The listing builds one solid part. Answer for the finished solid, in the listing's coordinates (mm). Face numbers are marked on the shaded views. A direction names the side the tool comes from. Round coordinates to 2 decimals unless told otherwise and drop trailing zeros. Order: outer loops, then holes, each group sorted by start corner. A loop starts at its lowest first (then second) coordinate and runs counter-clockwise, first axis right, second up. Notation, with made-up numbers: (42, 60) - (85, 60) arc R23 cw to (85, 95) - close; hole circle Ø5 at (44.5, 24). An arc over 180 degrees is marked (long way). Write item = value, one per line.
from build123d import *

# Parameters (mm, degrees)
SKETCH1_W           = 50
SKETCH1_H           = 25
BOSS_EXTRUDE1_DEPTH = 6
SKETCH2_R           = 1
SKETCH2_R_2         = 0.999812185
CUT_EXTRUDE1_DEPTH  = 6
CUT_EXTRUDE2_DEPTH  = 6
FILLET1_R           = 2


with BuildPart() as part:
    # Sketch1 → Boss-Extrude1 (new body)
    with BuildSketch(Plane(origin=(0, 0, 0), x_dir=(1, 0, 0), z_dir=(0, 1, 0))):
        Rectangle(SKETCH1_W, SKETCH1_H)
    extrude(amount=BOSS_EXTRUDE1_DEPTH)

    # Sketch2 → Cut-Extrude1 (cut)
    with BuildSketch(Plane(origin=(0, 0, 0), x_dir=(1, 0, 0), z_dir=(0, 1, 0))):
        with Locations((-21, 8.5)):
            Circle(SKETCH2_R)
        with Locations((21, 8.5)):
            Circle(SKETCH2_R_2)
        with Locations((-21, -8.5)):
            Circle(SKETCH2_R)
        with Locations((21, -8.5)):
            Circle(SKETCH2_R)
    extrude(amount=CUT_EXTRUDE1_DEPTH, mode=Mode.SUBTRACT)

    # Sketch3 → Cut-Extrude2 (cut)
    with BuildSketch(Plane(origin=(0, 0, 0), x_dir=(1, 0, 0), z_dir=(0, 1, 0))):
        Polygon((-22.5, 5.75), (-22.5, -5.75), (-18.25, -5.75), (-18.25, -10), (18.25, -10), (18.25, -5.75), (22.5, -5.75), (22.5, 5.75), (18.25, 5.75), (18.25, 10), (-18.25, 10), (-18.25, 5.75), align=None)
    extrude(amount=CUT_EXTRUDE2_DEPTH, mode=Mode.SUBTRACT)

    # Fillet1
    fillet1_edges = [part.edges().sort_by_distance(p)[0] for p in [
        (-18.25, 3, -5.75),
        (-18.25, 3, 5.75),
        (18.25, 3, 5.75),
        (18.25, 3, -5.75),
        (25, 3, 12.5),
        (-25, 3, 12.5),
        (-25, 3, -12.5),
        (25, 3, -12.5),
    ]]
    fillet(fillet1_edges, radius=FILLET1_R)


solid = part.part
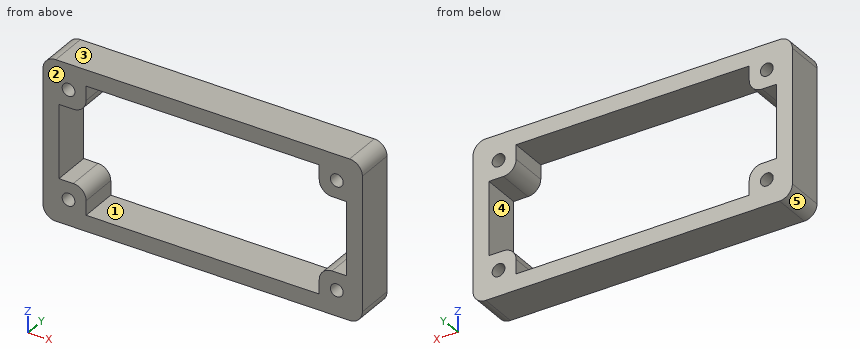
Q1. Section A-A on z = 2 is taken. Determine the outline of the cut face in (x, y).
Model answer:
outline = (-25, 0) - (-22.5, 0) - (-22.5, 6) - (-25, 6) - close; (22.5, 0) - (25, 0) - (25, 6) - (22.5, 6) - close
Q2. Section C-C on z = 8.5 is taken. Determine the outline of the cut face in (x, y).
Model answer:
outline = (-25, 0) - (-22, 0) - (-22, 6) - (-25, 6) - close; (-20, 0) - (-18.25, 0) - (-18.25, 6) - (-20, 6) - close; (18.25, 0) - (20, 0) - (20, 6) - (18.25, 6) - close; (22, 0) - (25, 0) - (25, 6) - (22, 6) - close
Q3. For the marked faces 1 and 2, determine the directions among +Z, -Z, +X, -X, +Y, -Y from which every point of the face is accessible in a straight line to the end or side of a thin tool.
Model answer:
face_1 = +Y, -Y
face_2 = +Z, -Z, +X, -X, -Y
Q4. Determine the mould class of the marked faces 3, 4 and 5 for opening direction Z: released by +Z, released by -Z, zero draft, split by the parting line, or undercut.
Model answer:
face_3 = released by +Z
face_4 = undercut
face_5 = released by -Z
Q5. Section D-D on x = -4 is taken. Determine the outline of the cut face in (y, z), then the cut area to 3 significant figures.
Model answer:
outline = (0, -12.5) - (6, -12.5) - (6, -10) - (0, -10) - close; (0, 10) - (6, 10) - (6, 12.5) - (0, 12.5) - close
area = 30.0 mm^2
Q6. Find the intervals of material crossed by line 1 (X direction, y = 3.9, z = -8.5); line 2 (Z direction, x = -21, y = 3.7); line 3 (Z direction, x = -11, y = 5.1), in increasing order. Write a range as from..to.
Model answer:
line_1 = -25..-22, -20..-18.25, 18.25..20, 22..25
line_2 = -12.5..-9.5, -7.5..-5.75, 5.75..7.5, 9.5..12.5
line_3 = -12.5..-10, 10..12.5
Q7. Section B-B on x = 21 is taken. Determine the outline of the cut face in (y, z), then the cut area to 3 significant figures.
Model answer:
outline = (0, -12.5) - (6, -12.5) - (6, -9.5) - (0, -9.5) - close; (0, -7.5) - (6, -7.5) - (6, -5.75) - (0, -5.75) - close; (0, 5.75) - (6, 5.75) - (6, 7.5) - (0, 7.5) - close; (0, 9.5) - (6, 9.5) - (6, 12.5) - (0, 12.5) - close
area = 57.0 mm^2
